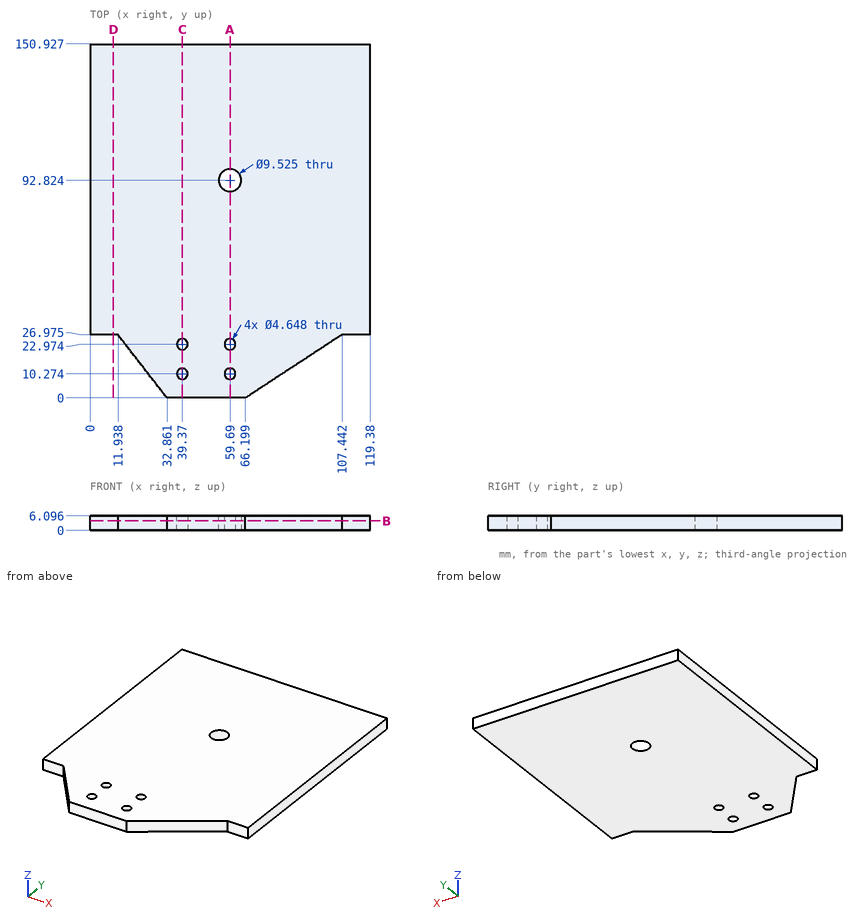
Study the drawing (mm; zero at the part's minimum x, y, z) and answer. Give positions to 0.01 mm unless a question says otherwise; leave off trailing zeros. Order: outer loops, then holes, each group sorted by start corner. A loop starts at its lowest first (then second) coordinate and runs counter-clockwise, first axis right, second up.
1. Section D-D, the plane x = 10 is taken. Determine the outline of the cut face in (y, z) (1 decimal).
Result sheet:
outline: (27, 0) - (150.9, 0) - (150.9, 6.1) - (27, 6.1) - close
2. Section A-A, the plane x = 59.69 is taken. Determine the outline of the cut face in (y, z).
Result sheet:
outline: (0, 0) - (7.95, 0) - (7.95, 6.1) - (0, 6.1) - close; (12.6, 0) - (20.65, 0) - (20.65, 6.1) - (12.6, 6.1) - close; (25.3, 0) - (88.06, 0) - (88.06, 6.1) - (25.3, 6.1) - close; (97.59, 0) - (150.93, 0) - (150.93, 6.1) - (97.59, 6.1) - close
3. Straight lines are drawn through the part: L1, parallel to Y at x = 60, z = 4.75; L2, parallel to Y at x = 39.5, z = 3.25 (1 decimal); L3, parallel to X at y = 9, z = 3.5 (1 decimal). For each, find the intervals that lie inside material, in ascending order.
Result sheet:
L1: y = 0 to 7.97, 12.58 to 20.67, 25.28 to 88.07, 97.58 to 150.93
L2: y = 0 to 8, 12.6 to 20.7, 25.3 to 150.9
L3: x = 25.9 to 37.4, 41.3 to 57.7, 61.6 to 80
4. Section B-B, the plane z = 4 is taken. Determine the outline of the cut face in (x, y) (1 decimal), and give its area (3 significant figures).
Result sheet:
outline: (0, 27) - (11.9, 27) - (32.9, 0) - (66.2, 0) - (107.4, 27) - (119.4, 27) - (119.4, 150.9) - (0, 150.9) - close; hole circle Ø4.6 at (39.4, 10.3); hole circle Ø4.6 at (39.4, 23); hole circle Ø9.5 at (59.7, 92.8); hole circle Ø4.6 at (59.7, 10.3); hole circle Ø4.6 at (59.7, 23)
area: 16,400 mm2
5. Each of these flat-tipped pins is pushed along its axis until it touches: P1, Ø3, axis at x = 59.69, y = 10.27, coming from the -Z side; P2, Ø6, axis at x = 59.69, y = 22.97, coming from the +Z side. Where does it stop, or does it pass through?
Result sheet:
P1: passes through
P2: stops at z = 6.1
6. Section C-C, the plane x = 39.37 is taken. Determine the outline of the cut face in (y, z).
Result sheet:
outline: (0, 0) - (7.95, 0) - (7.95, 6.1) - (0, 6.1) - close; (12.6, 0) - (20.65, 0) - (20.65, 6.1) - (12.6, 6.1) - close; (25.3, 0) - (150.93, 0) - (150.93, 6.1) - (25.3, 6.1) - close
